```python
from build123d import *

# Parameters (mm, degrees)
SKETCH1_R              = 1.7145
SKETCH1_R_2            = 2.8575
BASE_DEPTH             = 1.6002
SKETCH3_W              = 6.35
SKETCH3_H              = 69.255343758
BREADBOARD_SLICE_DEPTH = 0.8001
RPI_HOLES_SIZING_R     = 1.35
RPI_HOLES_DEPTH        = 157.444245717
WALL_BASE_W            = 76.5556
WALL_BASE_H            = 105.537
WALL_BASE_W_2          = 71.4756
WALL_BASE_H_2          = 100.457
WALL_DEPTH             = 76.2
USBC_DEPTH             = 2.54


with BuildPart() as part:
    # Sketch1 → Base (new body)
    with BuildSketch(Plane(origin=(0, 0, 0), x_dir=(1, 0, 0), z_dir=(0, 1, 0))):
        with BuildLine():
            Line((0, 22.5679), (0, 88.0491))
            ThreePointArc((0, 88.0491), (0.461248241, 89.162651759), (1.5748, 89.6239))
            Line((1.5748, 89.6239), (6.0579, 89.6239))
            ThreePointArc((6.0579, 89.6239), (12.020790064, 92.093809936), (14.4907, 98.0567))
            Line((14.4907, 98.0567), (14.4907, 109.0422))
            ThreePointArc((14.4907, 109.0422), (14.951948241, 110.155751759), (16.0655, 110.617))
            Line((16.0655, 110.617), (94.5515, 110.617))
            ThreePointArc((94.5515, 110.617), (95.665051759, 110.155751759), (96.1263, 109.0422))
            Line((96.1263, 109.0422), (96.1263, 98.0567))
            ThreePointArc((96.1263, 98.0567), (98.596209936, 92.093809936), (104.5591, 89.6239))
            Line((104.5591, 89.6239), (109.0422, 89.6239))
            ThreePointArc((109.0422, 89.6239), (110.155751759, 89.162651759), (110.617, 88.0491))
            Line((110.617, 88.0491), (110.617, 22.5679))
            ThreePointArc((110.617, 22.5679), (110.155751759, 21.454348241), (109.0422, 20.9931))
            Line((109.0422, 20.9931), (104.5591, 20.9931))
            ThreePointArc((104.5591, 20.9931), (98.596209936, 18.523190064), (96.1263, 12.5603))
            Line((96.1263, 12.5603), (96.1263, 1.5748))
            ThreePointArc((96.1263, 1.5748), (95.665051759, 0.461248241), (94.5515, 0))
            Line((94.5515, 0), (16.0655, 0))
            ThreePointArc((16.0655, 0), (14.951948241, 0.461248241), (14.4907, 1.5748))
            Line((14.4907, 1.5748), (14.4907, 12.5603))
            ThreePointArc((14.4907, 12.5603), (12.020790064, 18.523190064), (6.0579, 20.9931))
            Line((6.0579, 20.9931), (1.5748, 20.9931))
            ThreePointArc((1.5748, 20.9931), (0.461248241, 21.454348241), (0, 22.5679))
        make_face()
        with Locations(Location((6.0579, 83.312, 0), (0, 0, 270))):
            Circle(SKETCH1_R, mode=Mode.SUBTRACT)
        with Locations(Location((6.0579, 27.305, 0), (0, 0, 270))):
            Circle(SKETCH1_R, mode=Mode.SUBTRACT)
        with Locations(Location((6.0579, 55.3085, 0), (0, 0, 270))):
            Circle(SKETCH1_R, mode=Mode.SUBTRACT)
        with Locations(Location((104.5591, 83.312, 0), (0, 0, 270))):
            Circle(SKETCH1_R, mode=Mode.SUBTRACT)
        with Locations(Location((104.5591, 55.3085, 0), (0, 0, 270))):
            Circle(SKETCH1_R, mode=Mode.SUBTRACT)
        with Locations(Location((104.5591, 27.305, 0), (0, 0, 270))):
            Circle(SKETCH1_R, mode=Mode.SUBTRACT)
        with Locations(Location((6.0579, 74.3077, 0), (0, 0, 270))):
            Circle(SKETCH1_R_2, mode=Mode.SUBTRACT)
        with Locations(Location((104.5591, 74.3077, 0), (0, 0, 270))):
            Circle(SKETCH1_R_2, mode=Mode.SUBTRACT)
        with Locations(Location((104.5591, 36.3093, 0), (0, 0, 270))):
            Circle(SKETCH1_R_2, mode=Mode.SUBTRACT)
        with Locations(Location((6.0579, 36.3093, 0), (0, 0, 270))):
            Circle(SKETCH1_R_2, mode=Mode.SUBTRACT)
    extrude(amount=BASE_DEPTH)

    # Sketch3 → Breadboard Slice (cut)
    with BuildSketch(Plane(origin=(0, 1.6002, 0), x_dir=(1, 0, 0), z_dir=(0, 1, 0))):
        with Locations((86.546861599, 55.3085)):
            Rectangle(SKETCH3_W, SKETCH3_H)
    extrude(amount=-BREADBOARD_SLICE_DEPTH, mode=Mode.SUBTRACT)

    # RPi Holes + Sizing → RPi Holes (cut, through all)
    with BuildSketch(Plane(origin=(0, 1.6002, 0), x_dir=(1, 0, 0), z_dir=(0, 1, 0))):
        with Locations(Location((27.525509773, 93.558267586, 0), (0, 0, 270))):
            Circle(RPI_HOLES_SIZING_R)
        with Locations(Location((76.525509773, 93.558267586, 0), (0, 0, 270))):
            Circle(RPI_HOLES_SIZING_R)
        with Locations(Location((27.525509773, 35.558267586, 0), (0, 0, 270))):
            Circle(RPI_HOLES_SIZING_R)
        with Locations(Location((76.525509773, 35.558267586, 0), (0, 0, 270))):
            Circle(RPI_HOLES_SIZING_R)
    extrude(amount=-RPI_HOLES_DEPTH, mode=Mode.SUBTRACT)

    # Wall Base → Wall (add)
    with BuildSketch(Plane(origin=(0, 1.6002, 0), x_dir=(1, 0, 0), z_dir=(0, 1, 0))):
        with Locations((55.3085, 55.3085)):
            Rectangle(WALL_BASE_W, WALL_BASE_H)
        with Locations((55.3085, 55.3085)):
            Rectangle(WALL_BASE_W_2, WALL_BASE_H_2, mode=Mode.SUBTRACT)
    extrude(amount=WALL_DEPTH)

    # Sketch6 → USBC (cut)
    with BuildSketch(Plane.ZY.offset(-17.0307)):
        with BuildLine():
            Line((-85.633722135, 3.1002), (-78.783322135, 3.1002))
            ThreePointArc((-78.783322135, 3.1002), (-77.669770376, 3.561448241), (-77.208522135, 4.675))
            Line((-77.208522135, 4.675), (-77.208522135, 5.0254))
            ThreePointArc((-77.208522135, 5.0254), (-77.669770376, 6.138951759), (-78.783322135, 6.6002))
            Line((-78.783322135, 6.6002), (-85.633722135, 6.6002))
            ThreePointArc((-85.633722135, 6.6002), (-86.747273894, 6.138951759), (-87.208522135, 5.0254))
            Line((-87.208522135, 5.0254), (-87.208522135, 4.675))
            ThreePointArc((-87.208522135, 4.675), (-86.747273894, 3.561448241), (-85.633722135, 3.1002))
        make_face()
    extrude(amount=-USBC_DEPTH, mode=Mode.SUBTRACT)


solid = part.part
```
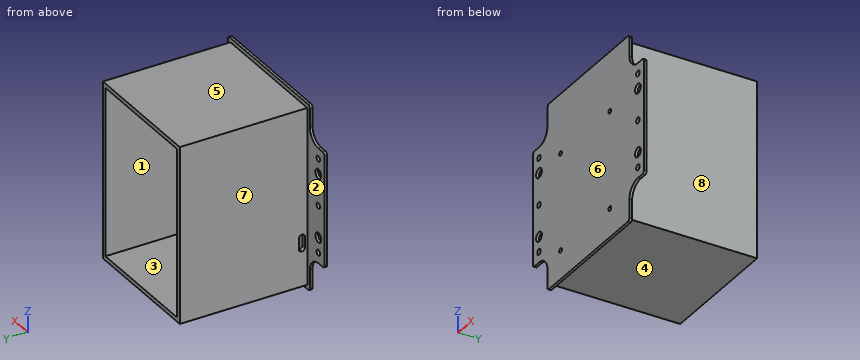
For this review, take the finished solid that the model builds, in its own axes (mm). Face numbers are marked on the shaded views. A direction names the side the tool comes from. Round coordinates to 2 decimals unless told otherwise and drop trailing zeros. Loops run counter-clockwise (first coordinate to the right, second up) from the corner with the lowest first, then second, coordinate; pieces in that order, holes last.
Q1. Machinability: for the marked faces 5, 6, 7 and 8, which of the approach directions +Z, -Z, +X, -X, +Y, -Y give a long, thin tool a straight path to every point of the face, cutting with its end or side? Answer none if there is none.
Result sheet:
face 5: +Z, +X, -X, +Y
face 6: +Z, -Z, +X, -X, -Y
face 7: +Z, -Z, -X, +Y
face 8: +Z, -Z, +X, +Y
Q2. Add section C-C on x = 38. Write out the cut boundary in (y, z), plus the area to 3 significant figures.
Result sheet:
outline: (0, -110.62) - (1.6, -110.62) - (1.6, -108.08) - (77.8, -108.08) - (77.8, -105.54) - (1.6, -105.54) - (1.6, -5.08) - (77.8, -5.08) - (77.8, -2.54) - (1.6, -2.54) - (1.6, 0) - (0, 0) - close
area: 564 mm2
Q3. Mouldability with a two-part tool opening along Z and no side actions: class the marked faces 1, 2, 3 and 4 as +Z half, -Z half, draft (parallel to the pull), parting line (faces both ways), or undercut.
Result sheet:
face 1: undercut
face 2: draft
face 3: undercut
face 4: -Z half
Q4. Add section A-A on y = 10.5. Write out the cut boundary in (x, z).
Result sheet:
outline: (17.03, -108.08) - (93.59, -108.08) - (93.59, -2.54) - (17.03, -2.54) - close; hole (19.57, -105.54) - (91.05, -105.54) - (91.05, -5.08) - (19.57, -5.08) - close
Q5. To check wall thickness, follow line 1 along Z through (x, y) = (71.5, 17); line 2 along X through (y, z) = (35, -95); line 3 along Y through (x, z) = (86, -71). State the ranges of each line that lie inside material, in increasing order.
Result sheet:
line 1: z = -108.08 to -105.54, -5.08 to -2.54
line 2: x = 17.03 to 19.57, 91.05 to 93.59
line 3: y = 0 to 0.8
Q6. Insertion check: pin 1 Ø1 at (y, z) = (48, -77) entering from +X; pin 2 Ø0.5 at (x, y) = (4, 1) entering from +Z; pin 3 Ø10 at (y, z) = (33.5, -39.5) entering from -X; pin 4 Ø3.5 at (x, z) = (104.56, -36.31) entering from -Y. Each pin has a flat end and moves straight along its axis. Give the tip position at first contact, or say it passes through.
Result sheet:
pin 1: stops at x = 93.59
pin 2: stops at z = -20.99
pin 3: stops at x = 17.03
pin 4: passes through
Q7. Add section D-D on z = -7. Write out the cut boundary in (x, y), plus the area to 3 significant figures.
Result sheet:
outline: (14.49, 0) - (96.13, 0) - (96.13, 1.6) - (93.59, 1.6) - (93.59, 77.8) - (91.05, 77.8) - (91.05, 1.6) - (19.57, 1.6) - (19.57, 77.8) - (17.03, 77.8) - (17.03, 1.6) - (14.49, 1.6) - close
area: 518 mm2
Q8. Add section B-B on z = -63.5. Write out the cut boundary in (x, y), plus the area to 3 significant figures.
Result sheet:
outline: (0, 0) - (110.62, 0) - (110.62, 1.6) - (93.59, 1.6) - (93.59, 77.8) - (91.05, 77.8) - (91.05, 1.6) - (89.72, 1.6) - (89.72, 0.8) - (83.37, 0.8) - (83.37, 1.6) - (19.57, 1.6) - (19.57, 77.8) - (17.03, 77.8) - (17.03, 1.6) - (0, 1.6) - close
area: 559 mm2
